CAD build for the part. Positions are in the model's coordinates, mm. A direction names the side the tool comes from. Coordinates: 2 decimals unless noted, no trailing zeros. Write each loop counter-clockwise with the first axis right and the second up, starting at its lowest first coordinate (ties: lowest second). Pieces come first, ordered by that corner, then holes. Notation, with made-up numbers: (4, 68.5) -> (15, 68.5) arc R24 ccw to (15, 87.5) -> close; hole circle Ø10 at (9.25, -38). An arc over 180 degrees is marked (long way). Answer as CSV lines item,"result". Start each with the question number.
```python
from build123d import *

# Parameters (mm, degrees)
F0_W     = 170
F0_H     = 530
F1_DEPTH = 250
F2_DEPTH = 15
F3_R     = 10
F4_DEPTH = 750


with BuildPart() as f1:
    # F0 (on Front) → F1 (new body)
    with BuildSketch(Plane.XZ):
        Polygon((100, 345), (100, 375), (-100, 375), (-100, -375), (100, -375), (100, -345), (15, -345), (15, -295), (100, -295), (100, 295), (15, 295), (15, 345), align=None)
        Rectangle(F0_W, F0_H, mode=Mode.SUBTRACT)
    extrude(amount=F1_DEPTH)

    # F0 (on Front) → F2 (join)
    with BuildSketch(Plane.XZ):
        Rectangle(F0_W, F0_H)
    extrude(amount=F2_DEPTH)

    # F3 (on face) → F4 (cut)
    with BuildSketch(Plane(origin=(0, 0, -375), x_dir=(1, 0, 0), z_dir=(0, 0, -1))):
        with Locations((50, 200)):
            Circle(F3_R)
        with Locations((50, 50)):
            Circle(F3_R)
    extrude(amount=-F4_DEPTH, mode=Mode.SUBTRACT)


solid = f1.part
```
1. Cut at A-A (y = -50). Count the separate pieces of the cut face and the enclosed holes in it, then the cut area to 3 significant figures.
2. Wall check: line 1 (Z direction, x = 21, y = -143); line 2 (Y direction, x = 50, z = -361.5); line 3 (X direction, y = -50, z = -354). Give the ranges that are in metal, low to high.
3. Tool access for faces 1 (the face through (-1, -131, -265)), 2 (the face through (15, -123, -320)), 3 (the face through (100, -123, -360)): list every direction of +Z, -Z, +X, -X, +Y, -Y with a clear straight run to the whole face (end or side of a thin tool).
4. Flat gauge pins, fed straight in: P1, Ø25, axis at y = -145.5, z = 325, coming from the +X side; P2, Ø12, axis at x = 50, y = -50, coming from the -Z side; P3, Ø1, axis at x = -41, z = -83.5, coming from the -Y side. Where does each tip first touch, or does it go through?
5. Mould opens along Y. For faces 4 (the face through (100, -123, 360)), 5 (the face through (-89, -250, 30)), 6 (the face through (47.83, -40.24, 359.79)), 7 (the face through (40, -200, -280)) say: pulls with the +Y half, pulls with the -Y half, needs draft (parallel to the pull), parting line crosses it, or undercut.
6. Cut at B-B (z = 172). Give the cut face in (x, y), then the cut area to 4 significant figures.
Geometry check:
1,separate pieces,"4"
1,enclosed holes,"0"
1,area,"49,000 mm²"
2,line 1,"-375 to -345, -295 to -265, 265 to 295, 345 to 375"
2,line 2,"-250 to -210, -190 to -60, -40 to 0"
2,line 3,"-100 to 40, 60 to 100"
3,face 1,"-Y"
3,face 2,"+X, +Y, -Y"
3,face 3,"+Z, -Z, +X, +Y, -Y"
4,P1,"x = 15"
4,P2,"through"
4,P3,"y = -15"
5,face 4,"needs draft"
5,face 5,"pulls with the -Y half"
5,face 6,"undercut"
5,face 7,"undercut"
6,outline,"(-100, -250) -> (-85, -250) -> (-85, -15) -> (85, -15) -> (85, -250) -> (100, -250) -> (100, 0) -> (-100, 0) -> close"
6,area,"10,050 mm²"
